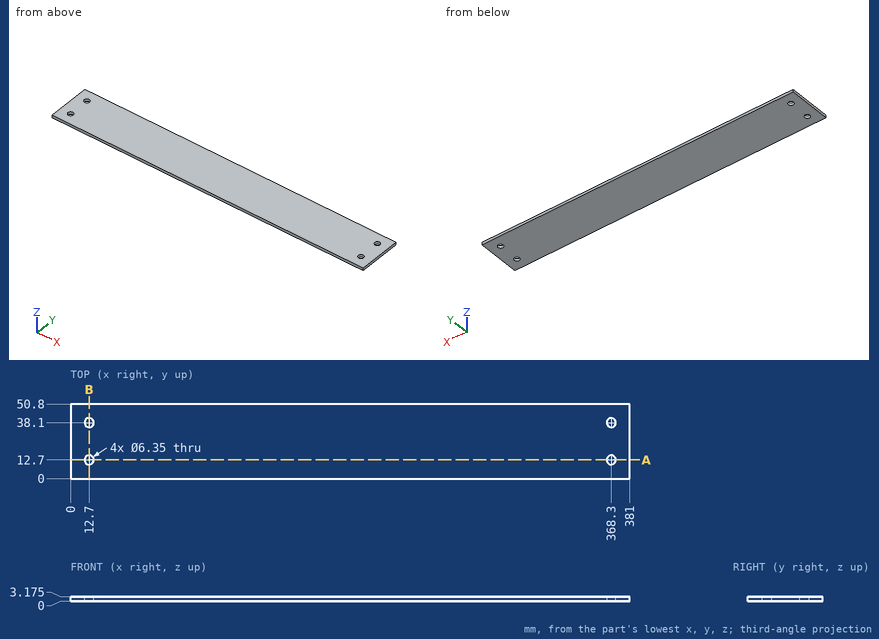
Verification items for this drawing (mm, ordinates from the low corner). Coordinates: 2 decimals unless noted, no trailing zeros. Loops run counter-clockwise (first coordinate to the right, second up) from the corner with the lowest first, then second, coordinate; pieces in that order, holes last. Notation, with made-up numbers: (47, 1.25) - (65, 1.25) arc R13 ccw to (65, 5.25) - close; hole circle Ø2 at (10.25, 65.5). An arc over 180 degrees is marked (long way). One line per item, written item: value. Start each with the question number.
(1) Material ranges on line 1 (Y direction, x = 368.3, z = 0.9) (3 decimals); line 2 (X direction, y = 10.5, z = 1.9); line 3 (X direction, y = 36, z = 1.25), recorded low to high. Write a range as [from, to].
(2) Depth check by flat-ended pin: P1, Ø4, axis at x = 368.3, y = 12.7, coming from the +Z side. Enter the tip coordinate at first touch or a pass-through.
(3) Cross-section at B-B on x = 12.7. Enter the section's corners in (y, z) (3 decimals), plus the area to 3 significant figures.
(4) Cross-section at A-A on y = 12.7. Enter the section's corners in (x, z) (3 decimals).
Results below:
1. line 1: y = [0, 9.525], [15.875, 34.925], [41.275, 50.8]
1. line 2: x = [0, 10.41], [14.99, 366.01], [370.59, 381]
1. line 3: x = [0, 10.32], [15.08, 365.92], [370.68, 381]
2. P1: passes through
3. outline: (0, 0) - (9.525, 0) - (9.525, 3.175) - (0, 3.175) - close; (15.875, 0) - (34.925, 0) - (34.925, 3.175) - (15.875, 3.175) - close; (41.275, 0) - (50.8, 0) - (50.8, 3.175) - (41.275, 3.175) - close
3. area: 121 mm2
4. outline: (0, 0) - (9.525, 0) - (9.525, 3.175) - (0, 3.175) - close; (15.875, 0) - (365.125, 0) - (365.125, 3.175) - (15.875, 3.175) - close; (371.475, 0) - (381, 0) - (381, 3.175) - (371.475, 3.175) - close
